```python
from build123d import *

# Parameters (mm, degrees)
SKETCH1_R           = 20.32
BOSS_EXTRUDE3_DEPTH = 10.16


with BuildPart() as part:
    # Sketch1 → Boss-Extrude3 (new body)
    with BuildSketch(Plane.XY):
        with BuildLine():
            Line((37.321963159, 51.023310491), (30.908331921, 55.145101009))
            ThreePointArc((30.908331921, 55.145101009), (28.995188409, 55.490270076), (27.398320271, 54.381544712))
            Line((27.398320271, 54.381544712), (21.905409565, 45.834408819))
            ThreePointArc((21.905409565, 45.834408819), (14.312013888, 48.74224306), (6.351949066, 50.401316878))
            Line((6.351949066, 50.401316878), (6.351949066, 60.561316878))
            ThreePointArc((6.351949066, 60.561316878), (5.608000291, 62.357368102), (3.811949066, 63.101316878))
            Line((3.811949066, 63.101316878), (-3.811949066, 63.101316878))
            ThreePointArc((-3.811949066, 63.101316878), (-5.608000291, 62.357368102), (-6.351949066, 60.561316878))
            Line((-6.351949066, 60.561316878), (-6.351949066, 50.401316878))
            ThreePointArc((-6.351949066, 50.401316878), (-14.312013888, 48.74224306), (-21.905409565, 45.834408819))
            Line((-21.905409565, 45.834408819), (-27.398320271, 54.381544712))
            ThreePointArc((-27.398320271, 54.381544712), (-28.995188409, 55.490270076), (-30.908331921, 55.145101009))
            Line((-30.908331921, 55.145101009), (-37.321963159, 51.023310491))
            ThreePointArc((-37.321963159, 51.023310491), (-38.430688522, 49.426442353), (-38.085519456, 47.513298841))
            Line((-38.085519456, 47.513298841), (-32.59260875, 38.966162948))
            ThreePointArc((-32.59260875, 38.966162948), (-38.392078377, 33.266925284), (-43.207955436, 26.71539981))
            Line((-43.207955436, 26.71539981), (-52.449816509, 30.936016342))
            ThreePointArc((-52.449816509, 30.936016342), (-54.392609658, 31.005403375), (-55.81543591, 29.680705207))
            Line((-55.81543591, 29.680705207), (-58.982517652, 22.745763536))
            ThreePointArc((-58.982517652, 22.745763536), (-59.051904686, 20.802970387), (-57.727206517, 19.380144135))
            Line((-57.727206517, 19.380144135), (-48.485345444, 15.159527603))
            ThreePointArc((-48.485345444, 15.159527603), (-50.282929248, 7.229593784), (-50.792280749, -0.885559877))
            Line((-50.792280749, -0.885559877), (-60.848866599, -2.331478634))
            ThreePointArc((-60.848866599, -2.331478634), (-62.520761661, -3.323459823), (-63.001533372, -5.207104785))
            Line((-63.001533372, -5.207104785), (-61.916539542, -12.753402628))
            ThreePointArc((-61.916539542, -12.753402628), (-60.924558353, -14.42529769), (-59.040913391, -14.906069401))
            Line((-59.040913391, -14.906069401), (-48.984327541, -13.460150644))
            ThreePointArc((-48.984327541, -13.460150644), (-46.209305364, -21.10308266), (-42.250415805, -28.20536056))
            Line((-42.250415805, -28.20536056), (-49.928831481, -34.858745616))
            ThreePointArc((-49.928831481, -34.858745616), (-50.799013587, -36.59714801), (-50.185089135, -38.441695799))
            Line((-50.185089135, -38.441695799), (-45.192497609, -44.203453568))
            ThreePointArc((-45.192497609, -44.203453568), (-43.454095215, -45.073635675), (-41.609547426, -44.459711223))
            Line((-41.609547426, -44.459711223), (-33.93113175, -37.806326166))
            ThreePointArc((-33.93113175, -37.806326166), (-27.464553527, -42.735679468), (-20.29434237, -46.570158554))
            Line((-20.29434237, -46.570158554), (-23.156745148, -56.318607166))
            ThreePointArc((-23.156745148, -56.318607166), (-22.948937628, -58.251500287), (-21.435233689, -59.471320013))
            Line((-21.435233689, -59.471320013), (-14.120156999, -61.619220327))
            ThreePointArc((-14.120156999, -61.619220327), (-12.187263879, -61.411412808), (-10.967444152, -59.897708869))
            Line((-10.967444152, -59.897708869), (-8.105041374, -50.149260257))
            ThreePointArc((-8.105041374, -50.149260257), (0, -50.8), (8.105041374, -50.149260257))
            Line((8.105041374, -50.149260257), (10.967444152, -59.897708869))
            ThreePointArc((10.967444152, -59.897708869), (12.187263879, -61.411412808), (14.120156999, -61.619220327))
            Line((14.120156999, -61.619220327), (21.435233689, -59.471320013))
            ThreePointArc((21.435233689, -59.471320013), (22.948937628, -58.251500287), (23.156745148, -56.318607166))
            Line((23.156745148, -56.318607166), (20.29434237, -46.570158554))
            ThreePointArc((20.29434237, -46.570158554), (27.464553527, -42.735679468), (33.93113175, -37.806326166))
            Line((33.93113175, -37.806326166), (41.609547426, -44.459711223))
            ThreePointArc((41.609547426, -44.459711223), (43.454095215, -45.073635675), (45.192497609, -44.203453568))
            Line((45.192497609, -44.203453568), (50.185089135, -38.441695799))
            ThreePointArc((50.185089135, -38.441695799), (50.799013587, -36.59714801), (49.928831481, -34.858745616))
            Line((49.928831481, -34.858745616), (42.250415805, -28.205360559))
            ThreePointArc((42.250415805, -28.205360559), (46.209305364, -21.10308266), (48.984327541, -13.460150644))
            Line((48.984327541, -13.460150644), (59.040913391, -14.906069401))
            ThreePointArc((59.040913391, -14.906069401), (60.924558353, -14.42529769), (61.916539542, -12.753402628))
            Line((61.916539542, -12.753402628), (63.001533372, -5.207104785))
            ThreePointArc((63.001533372, -5.207104785), (62.520761661, -3.323459823), (60.848866599, -2.331478634))
            Line((60.848866599, -2.331478634), (50.792280749, -0.885559877))
            ThreePointArc((50.792280749, -0.885559877), (50.282929248, 7.229593784), (48.485345444, 15.159527603))
            Line((48.485345444, 15.159527603), (57.727206517, 19.380144135))
            ThreePointArc((57.727206517, 19.380144135), (59.051904686, 20.802970387), (58.982517652, 22.745763536))
            Line((58.982517652, 22.745763536), (55.81543591, 29.680705207))
            ThreePointArc((55.81543591, 29.680705207), (54.392609658, 31.005403375), (52.449816509, 30.936016342))
            Line((52.449816509, 30.936016342), (43.207955436, 26.71539981))
            ThreePointArc((43.207955436, 26.71539981), (38.392078377, 33.266925284), (32.59260875, 38.966162948))
            Line((32.59260875, 38.966162948), (38.085519456, 47.513298841))
            ThreePointArc((38.085519456, 47.513298841), (38.430688522, 49.426442353), (37.321963159, 51.023310491))
        make_face()
        Circle(SKETCH1_R, mode=Mode.SUBTRACT)
    extrude(amount=BOSS_EXTRUDE3_DEPTH)


solid = part.part
```
For this review, take the finished solid that the model builds, in its own axes (mm). A direction names the side the tool comes from. Round coordinates to 2 decimals unless told otherwise and drop trailing zeros. Write each loop counter-clockwise with the first axis right and the second up, starting at its lowest first coordinate (ties: lowest second). Pieces come first, ordered by that corner, then holes. Notation, with made-up numbers: (79.25, 53.5) - (101.25, 53.5) arc R7 ccw to (101.25, 57.5) - close; hole circle Ø4 at (16.5, 79.25). An arc over 180 degrees is marked (long way). Answer as a JSON object with one key per item and string values.
1. We need section A-A on x = 0. Give the boundary of the cut face in (y, z), then the cut area to 3 significant figures.
Response values:
{"outline": "(-50.8, 0) - (-20.32, 0) - (-20.32, 10.16) - (-50.8, 10.16) - close; (20.32, 0) - (63.1, 0) - (63.1, 10.16) - (20.32, 10.16) - close", "area": "744 mm2"}
2. To check wall thickness, follow line 1 along Y through (x, z) = (0, 2.25); line 2 along Y through (x, z) = (56.5, 5.25); line 3 along X through (y, z) = (-0.5, 6.75). State the ranges of each line that lie inside material, in increasing order.
Response values:
{"line 1": "y = -50.8 to -20.32, 20.32 to 63.1", "line 2": "y = -14.54 to -1.71, 18.82 to 28.18", "line 3": "x = -50.8 to -20.31, 20.31 to 50.8"}
3. We need section C-C on y = -24.5. Give the boundary of the cut face in (x, z), then the cut area to 3 significant figures.
Response values:
{"outline": "(-44.5, 0) - (44.5, 0) - (44.5, 10.16) - (-44.5, 10.16) - close", "area": "904 mm2"}
4. We need section D-D on y = 43. Give the boundary of the cut face in (x, z) (3 decimals).
Response values:
{"outline": "(-35.185, 0) - (35.185, 0) - (35.185, 10.16) - (-35.185, 10.16) - close"}
5. We need section B-B on y = 9. Give the boundary of the cut face in (x, z), then the cut area to 3 significant figures.
Response values:
{"outline": "(-50, 0) - (-18.22, 0) - (-18.22, 10.16) - (-50, 10.16) - close; (18.22, 0) - (50, 0) - (50, 10.16) - (18.22, 10.16) - close", "area": "646 mm2"}
6. For pin 1 Ø4 at (x, z) = (-27.5, 7) entering from +Y; pin 2 Ø3 at (x, z) = (-33, 4) entering from +Y; pin 3 Ø5 at (y, z) = (57, 5.5) entering from -X, all flat-tipped, find the tip position at first contact; note any pin that passes through.
Response values:
{"pin 1": "stops at y = 55.55", "pin 2": "stops at y = 54.76", "pin 3": "stops at x = -31.91"}
7. Draft analysis for pull direction Y (two halves, no side actions). For faces 1 (the face through (46.143, -31.579, 5.009)), 2 (the face through (-46.257, -20.999, 5.009)), 3 (the face through (-0.1, -50.8, 5)), 4 (the face through (54.419, 30.995, 5.009)), state which applies: +Y half, -Y half, draft (parallel to the pull), parting line (faces both ways), or undercut.
Response values:
{"face 1": "undercut", "face 2": "undercut", "face 3": "-Y half", "face 4": "+Y half"}
8. Tool access review of faces 5 (the face through (50.3, 7.1, 5)), 6 (the face through (-24.613, 50.048, 5.009)), 7 (the face through (37.72, -41.09, 5.01)), 8 (the face through (-21.706, -51.376, 5.009)): name each direction out of +Z, -Z, +X, -X, +Y, -Y from which nothing blocks a thin tool from reaching the whole face with its end or side.
Response values:
{"face 5": "+Z, -Z, +X", "face 6": "+Z, -Z, +Y", "face 7": "+Z, -Z, -Y", "face 8": "+Z, -Z, -X"}
